```python
from build123d import *

# Parameters (mm, degrees)
SKETCH_1_W          = 100
SKETCH_1_H          = 20
SKETCH_1_W_2        = 15
SKETCH_1_H_2        = 120
EXTRUDE_1_DEPTH     = 10
SKETCH_1_3_W        = 15
SKETCH_1_3_H        = 120
EXTRUDE_2_DEPTH     = 15
SKETCH_2_R          = 1.6
CUT_EXTRUDE_1_DEPTH = 15
EXTRUDE_START       = 10
EXTRUDE_3_DEPTH     = 20
SKETCH_5_R          = 1.6
CUT_EXTRUDE_4_DEPTH = 100
SKETCH_6_R          = 1.6
CUT_EXTRUDE_5_DEPTH = 100
CUT_EXTRUDE_START   = -20
SKETCH_7_R          = 2.1
CUT_EXTRUDE_6_DEPTH = 100


with BuildPart() as part:
    # Sketch 1 → Extrude 1 (new body)
    with BuildSketch(Plane(origin=(0, 0, 0), x_dir=(1, 0, 0), z_dir=(0, 1, 0))):
        Polygon((-7.5, -10), (-50, -10), (-7.5, -130), align=None)
        Rectangle(SKETCH_1_W, SKETCH_1_H)
        with Locations((0, -70)):
            Rectangle(SKETCH_1_W_2, SKETCH_1_H_2)
        Polygon((50, -10), (7.5, -10), (7.5, -130), align=None)
    extrude(amount=EXTRUDE_1_DEPTH)

    # Sketch 1_3 → Extrude 2 (add)
    with BuildSketch(Plane(origin=(0, 0, 0), x_dir=(1, 0, 0), z_dir=(0, 1, 0))):
        Polygon((-7.5, -10), (-50, -10), (-7.5, -130), align=None)
        with Locations((0, -70)):
            Rectangle(SKETCH_1_3_W, SKETCH_1_3_H)
        Polygon((50, -10), (7.5, -10), (7.5, -130), align=None)
    extrude(amount=EXTRUDE_2_DEPTH)

    # Sketch 2 → Cut-Extrude 1 (cut)
    with BuildSketch(Plane(origin=(0, 10, 0), x_dir=(1, 0, 0), z_dir=(0, 1, 0))):
        with Locations(Location((20, 0, 0), (0, 0, 270))):
            Circle(SKETCH_2_R)
        with Locations(Location((-20, 0, 0), (0, 0, 270))):
            Circle(SKETCH_2_R)
    extrude(amount=-CUT_EXTRUDE_1_DEPTH, mode=Mode.SUBTRACT)

    # Sketch 1_4 → Extrude 3 (add)
    with BuildSketch(Plane(origin=(0, 0, 0), x_dir=(1, 0, 0), z_dir=(0, 1, 0)).offset(EXTRUDE_START)):
        Polygon((-7.5, -10), (-50, -10), (-7.5, -130), align=None)
        Polygon((50, -10), (7.5, -10), (7.5, -130), align=None)
    extrude(amount=EXTRUDE_3_DEPTH)

    # Sketch 5 → Cut-Extrude 4 (cut)
    with BuildSketch(Plane(origin=(0, 30, 0), x_dir=(1, 0, 0), z_dir=(0, 1, 0))):
        with Locations(Location((22, -40, 0), (0, 0, 270))):
            Circle(SKETCH_5_R)
        with Locations(Location((-22, -40, 0), (0, 0, 270))):
            Circle(SKETCH_5_R)
    extrude(amount=-CUT_EXTRUDE_4_DEPTH, mode=Mode.SUBTRACT)

    # Sketch 6 → Cut-Extrude 5 (cut)
    with BuildSketch(Plane(origin=(0, 0, 10), x_dir=(-1, 0, 0), z_dir=(0, 0, -1))):
        with Locations((40, 23)):
            Circle(SKETCH_6_R)
        with Locations((-40, 23)):
            Circle(SKETCH_6_R)
    extrude(amount=-CUT_EXTRUDE_5_DEPTH, mode=Mode.SUBTRACT)

    # Sketch 7 → Cut-Extrude 6 (cut)
    with BuildSketch(Plane(origin=(0, 0, 10), x_dir=(-1, 0, 0), z_dir=(0, 0, -1)).offset(CUT_EXTRUDE_START)):
        with Locations((-40, 23)):
            Circle(SKETCH_7_R)
        with Locations((40, 23)):
            Circle(SKETCH_7_R)
    extrude(amount=-CUT_EXTRUDE_6_DEPTH, mode=Mode.SUBTRACT)


solid = part.part
```
Can you work these out from the model? Positions are in its coordinate system, mm. A direction names the side the tool comes from. Coordinates: 2 decimals unless noted, no trailing zeros. Loops run counter-clockwise (first coordinate to the right, second up) from the corner with the lowest first, then second, coordinate; pieces in that order, holes last. Notation, with made-up numbers: (48.5, 49) -> (68.5, 49) arc R24 cw to (68.5, 77) -> close; hole circle Ø2 at (-25.5, -31.5). An arc over 180 degrees is marked (long way). Put each result on its own line as item: value. Start each with the question number.
Q1. If I drill on line 1 (X direction, y = 4.5, z = 0); line 2 (X direction, y = 21.5, z = 31); line 3 (X direction, y = 13.5, z = 40) (3 decimals), over which ranges is the centre line in solid material (lowest first)? Write a range as [from, to].
Q2. For faces 4 (the face through (-7.5, 22, 71)), 5 (the face through (-20, 30, 42)), 6 (the face through (1, 13, 10)), which set-ups out of +Z, -Z, +X, -X, +Y, -Y let a thin tool reach every point of the face, with its end or its side?
Q3. I'm going to push flat-ended pins straight in: P1, Ø3.5, axis at x = -20, z = 0, coming from the +Y side; P2, Ø2.5, axis at x = -40, y = 23, coming from the -Z side; P3, Ø8, axis at y = 12.5, z = 33.5, coming from the -X side; P4, Ø7.5, axis at y = 25, z = 51, coming from the -X side. Where does each tip first touch, or does it pass through?
Q4. I want a section at A-A (y = 18.25). Write out the boundary of the cut face in (x, z), plus the area to 3 significant figures.
Q5. I want a section at D-D (z = 96.5). Write out the boundary of the cut face in (x, y).
Q6. I want a section at B-B (z = 0). Write out the boundary of the cut face in (x, y), plus the area to 3 significant figures.
Q7. Thinking about a two-plate mould opening in Y: for faces 1 (the face through (21.586, 5.07, -0.208)), 2 (the face through (-1, 10, 0)), 3 (the face through (40.208, 24.586, 19.86)), which applies, pulls with the +Y half, pulls with the -Y half, needs draft (parallel to the pull), parting line crosses it, or undercut?
Q8. I want a section at C-C (x = -1). Write out the boundary of the cut face in (y, z).
Taken from the geometry:
1. line 1: x = [-50, -21.6], [-18.4, 18.4], [21.6, 50]
1. line 2: x = [-42.56, -41.47], [-38.53, -7.5], [7.5, 38.53], [41.47, 42.56]
1. line 3: x = [-39.375, -23.6], [-20.4, 20.4], [23.6, 39.375]
2. face 4: +Z, -Z, +Y
2. face 5: +Z, -Z, +X, -X, +Y
2. face 6: -Z, +X, -X, +Y
3. P1: stops at y = 10
3. P2: passes through
3. P3: stops at x = -43.09
3. P4: stops at x = -36.81
4. outline: (-50, 10) -> (-7.5, 10) -> (-7.5, 130) -> close; (7.5, 10) -> (50, 10) -> (7.5, 130) -> close; hole circle Ø3.2 at (-22, 40); hole circle Ø3.2 at (22, 40)
4. area: 5,080 mm2
5. outline: (-19.36, 0) -> (19.36, 0) -> (19.36, 30) -> (7.5, 30) -> (7.5, 15) -> (-7.5, 15) -> (-7.5, 30) -> (-19.36, 30) -> close
6. outline: (-50, 0) -> (-21.6, 0) -> (-21.6, 10) -> (-50, 10) -> close; (-18.4, 0) -> (18.4, 0) -> (18.4, 10) -> (-18.4, 10) -> close; (21.6, 0) -> (50, 0) -> (50, 10) -> (21.6, 10) -> close
6. area: 936 mm2
7. face 1: needs draft
7. face 2: pulls with the +Y half
7. face 3: undercut
8. outline: (0, -10) -> (10, -10) -> (10, 10) -> (15, 10) -> (15, 130) -> (0, 130) -> close
